```python
from build123d import *

# Parameters (mm, degrees)
F1_DEPTH = 25


# Not quite as in the source:
# - ends of sketch curves that miss each other by under 0.0002 mm in the source are joined


with BuildPart() as f1:
    # F0 (on Top) → F1 (new body)
    with BuildSketch(Plane.XY):
        with BuildLine():
            Line((-7.9011580417, 39.7218038563), (0, 0))
            Line((0, 0), (0, 40.5))
            ThreePointArc((0, 40.5), (-0.0234209669, 40.4999932279), (-0.046841926, 40.4999729115))
            ThreePointArc((-0.046841926, 40.4999729115), (-3.9930017081, 40.3026790345), (-7.9011580417, 39.7218038563))
        make_face()
        with BuildLine():
            Line((-15.4986790108, 37.4171210667), (0, 0))
            Line((0, 0), (-7.9011580417, 39.7218038563))
            ThreePointArc((-7.9011580417, 39.7218038563), (-11.7565294288, 38.7560835972), (-15.4986790108, 37.4171210667))
        make_face()
        with BuildLine():
            Line((22.5005944373, 33.6745192983), (0, 0))
            Line((0, 0), (28.6378246381, 28.6378246381))
            ThreePointArc((28.6378246381, 28.6378246381), (25.6929280086, 31.3069233612), (22.5005944373, 33.6745192983))
        make_face()
        with BuildLine():
            Line((15.4986790108, 37.4171210667), (0, 0))
            Line((0, 0), (22.5005944373, 33.6745192983))
            ThreePointArc((22.5005944373, 33.6745192983), (19.1122200978, 35.7067646663), (15.5419449411, 37.3991704112))
            ThreePointArc((15.5419449411, 37.3991704112), (15.5203145712, 37.4081519941), (15.4986790108, 37.4171210667))
        make_face()
        with BuildLine():
            Line((7.9011580417, 39.7218038563), (0, 0))
            Line((0, 0), (15.4986790108, 37.4171210667))
            ThreePointArc((15.4986790108, 37.4171210667), (11.7565294288, 38.7560835972), (7.9011580417, 39.7218038563))
        make_face()
        with BuildLine():
            Line((0, 40.5), (0, 0))
            Line((0, 0), (7.9011580417, 39.7218038563))
            ThreePointArc((7.9011580417, 39.7218038563), (3.9696941833, 40.3049814302), (0, 40.5))
        make_face()
        with BuildLine():
            add(Edge.make_bspline(
                [(0, 40.5), (2.7706806954, 40.5108669818), (5.5531529278, 41.2084422704), (8.0962483637, 40.7025891367)],
                knots=[0.375, 0.375, 0.375, 0.375, 0.5, 0.5, 0.5, 0.5], degree=3))
            ThreePointArc((0, 40.5), (3.9696941833, 40.3049814302), (7.9011580417, 39.7218038563))
            Line((7.9011580417, 39.7218038563), (8.0962483637, 40.7025891367))
        make_face()
        with BuildLine():
            ThreePointArc((-15.4986790108, 37.4171210667), (-11.7565294288, 38.7560835972), (-7.9011580417, 39.7218038563))
            Line((-7.9011580417, 39.7218038563), (-8.0962483637, 40.7025891367))
            ThreePointArc((-8.0962483637, 40.7025891367), (-8.3021528679, 40.6610902185), (-8.5078446962, 40.6185496864))
            add(Edge.make_bspline(
                [(-15.4986790108, 37.4171210667), (-13.169476805, 38.5739896459), (-10.9180232176, 40.0695028236), (-8.5078446962, 40.6185496864)],
                knots=[0.125, 0.125, 0.125, 0.125, 0.2432920147, 0.2432920147, 0.2432920147, 0.2432920147], degree=3))
        make_face()
        with BuildLine():
            Line((-8.0962483637, 40.7025891367), (-7.9011580417, 39.7218038563))
            ThreePointArc((-7.9011580417, 39.7218038563), (-3.9930017081, 40.3026790345), (-0.046841926, 40.4999729115))
            add(Edge.make_bspline(
                [(-8.0962483637, 40.7025891367), (-5.5440345136, 41.1623685455), (-2.801770338, 40.4967143515), (-0.046841926, 40.4999729115)],
                knots=[0.25, 0.25, 0.25, 0.25, 0.3742955555, 0.3742955555, 0.3742955555, 0.3742955555], degree=3))
        make_face()
        with BuildLine():
            ThreePointArc((22.5005944373, 33.6745192983), (25.6929280086, 31.3069233612), (28.6378246381, 28.6378246381))
            add(Edge.make_bspline(
                [(23.4042695923, 34.2708354852), (25.4208730599, 32.841246937), (26.9286368317, 30.597978935), (28.6378246381, 28.6378246381)],
                knots=[0.7567079853, 0.7567079853, 0.7567079853, 0.7567079853, 0.875, 0.875, 0.875, 0.875], degree=3))
            ThreePointArc((23.4042695923, 34.2708354852), (23.230514679, 34.388852667), (23.0561646703, 34.5059889106))
            Line((23.0561646703, 34.5059889106), (22.5005944373, 33.6745192983))
        make_face()
        with BuildLine():
            ThreePointArc((15.5419449411, 37.3991704112), (19.1122200978, 35.7067646663), (22.5005944373, 33.6745192983))
            Line((22.5005944373, 33.6745192983), (23.0561646703, 34.5059889106))
            add(Edge.make_bspline(
                [(15.5419449411, 37.3991704112), (18.0859199176, 36.3418944337), (20.8741764939, 35.907459652), (23.0561646703, 34.5059889106)],
                knots=[0.6257044445, 0.6257044445, 0.6257044445, 0.6257044445, 0.75, 0.75, 0.75, 0.75], degree=3))
        make_face()
        with BuildLine():
            ThreePointArc((7.9011580417, 39.7218038563), (11.7565294288, 38.7560835972), (15.4986790108, 37.4171210667))
            add(Edge.make_bspline(
                [(8.0962483637, 40.7025891367), (10.6393437996, 40.1967360031), (12.9430624391, 38.4874544473), (15.4986790108, 37.4171210667)],
                knots=[0.5, 0.5, 0.5, 0.5, 0.625, 0.625, 0.625, 0.625], degree=3))
            Line((8.0962483637, 40.7025891367), (7.9011580417, 39.7218038563))
        make_face()
    extrude(amount=F1_DEPTH)


solid = f1.part
```
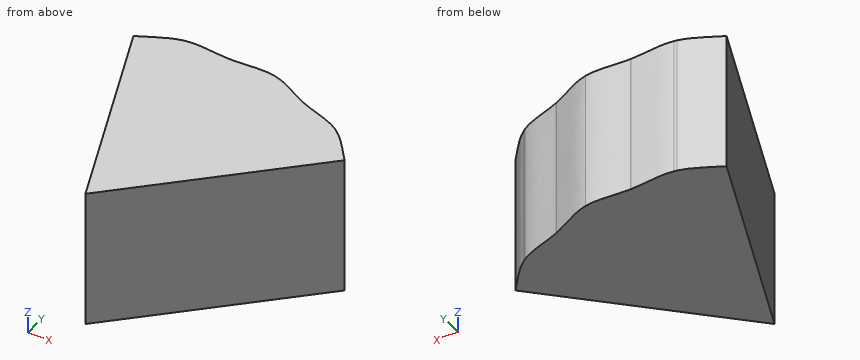
Build history of the part. All positions in model axes, mm. Round coordinates to 2 decimals unless told otherwise and drop trailing zeros. Loops run counter-clockwise (first coordinate to the right, second up) from the corner with the lowest first, then second, coordinate; pieces in that order, holes last.
Item 1: Drill centre lines: line 1 along X through (y, z) = (28, 15); line 2 along X through (y, z) = (18, 23.75); line 3 along Y through (x, z) = (12, 16.5). Where is each one in solid material? Low to high.
Item 2: Saw through at A-A (y = 21). List the corners of the cut face in (x, z).
Item 3: Pin check, flat tips, straight feed: P1, Ø3, axis at y = 23, z = 6, coming from the +X side; P2, Ø1, axis at y = 11, z = 17, coming from the -X side; P3, Ø4, axis at y = 16.5, z = 4, coming from the +X side. Stop position of each tip, or through.
Item 4: Saw through at B-B (y = 5). List the corners of the cut face in (x, z), then the cut area to 3 significant figures.
Worked answers:
1. line 1: x = -11.6 to 28
1. line 2: x = -7.46 to 18
1. line 3: y = 12 to 39.16
2. outline: (-8.7, 0) - (21, 0) - (21, 25) - (-8.7, 25) - close
3. P1: stops at x = 24.5
3. P2: stops at x = -4.76
3. P3: stops at x = 18.5
4. outline: (-2.07, 0) - (5, 0) - (5, 25) - (-2.07, 25) - close
4. area: 177 mm2
